Here's how the part is built. I have some questions about the finished solid (model axes, mm). A direction names the side the tool comes from. Coordinates: 2 decimals unless noted, no trailing zeros. Write each loop counter-clockwise with the first axis right and the second up, starting at its lowest first coordinate (ties: lowest second). Pieces come first, ordered by that corner, then holes. Notation, with made-up numbers: (59, 18.25) -> (67, 18.25) arc R17 ccw to (67, 34.25) -> close; hole circle Ø10 at (31.5, 13). An arc over 180 degrees is marked (long way). Put each result on its own line as item: value.
```python
from build123d import *

# Parameters (mm, degrees)
PAD_DEPTH            = 31
FILLET_R             = 15
POCKET_DEPTH         = 24.023168
FILLET001_R          = 15
POCKET001_DEPTH      = 18.144337
POCKET001_DEPTH_BACK = -16.633037
FILLET002_R          = 10
SKETCH003_R          = 7.670171
POCKET002_DEPTH      = 18.144337
POCKET002_DEPTH_BACK = -16.633037
POCKET003_DEPTH      = 18.144337
POCKET003_DEPTH_BACK = -16.633037


with BuildPart() as part:
    # Sketch → Pad (new body)
    with BuildSketch(Plane.XY):
        with BuildLine():
            Line((17.5802, 5.874869), (-57.733299, 5.874869))
            Line((-57.733299, 5.874869), (-57.733299, -5.878831))
            Line((-57.733299, -5.878831), (17.914803, -5.878831))
            ThreePointArc((24.661976, -7.143267), (21.347118, -6.197668), (17.914803, -5.878831))
            Line((24.661976, -7.143267), (45.314852, -15.165812))
            ThreePointArc((45.314852, -15.165812), (49.158723, -16.262318), (53.138796, -16.632037))
            Line((53.138796, -16.632037), (98.306877, -16.632037))
            Line((98.306877, -16.632037), (98.306877, -11.884055))
            Line((98.306877, -11.884055), (53.335909, -11.884055))
            ThreePointArc((45.371277, -10.225885), (49.268204, -11.465115), (53.335909, -11.884055))
            Line((32.389291, -4.575495), (45.371277, -10.225885))
            ThreePointArc((32.39346, 4.595455), (29.384719, 0.011347), (32.389291, -4.575495))
            Line((44.784154, 9.975093), (32.39346, 4.595455))
            ThreePointArc((53.974339, 11.884055), (49.281162, 11.401775), (44.784154, 9.975093))
            Line((98.300218, 11.884055), (53.974339, 11.884055))
            Line((98.300218, 18.143337), (98.300218, 11.884055))
            Line((53.605767, 18.143337), (98.300218, 18.143337))
            ThreePointArc((53.605767, 18.143337), (50.367046, 17.81052), (47.2637, 16.825979))
            Line((26.131771, 7.651179), (47.2637, 16.825979))
            ThreePointArc((17.5802, 5.874869), (21.947254, 6.323636), (26.131771, 7.651179))
        make_face()
    extrude(amount=PAD_DEPTH)

    # Fillet
    fillet_edges = [part.edges().sort_by_distance(p)[0] for p in [
        (98.306877, -14.258046, 31),
        (98.300218, 15.013696, 31),
        (98.306877, -14.258046, 0),
        (98.300218, 15.013696, 0),
    ]]
    fillet(fillet_edges, radius=FILLET_R)

    # Sketch001 (on Face13 of Fillet) → Pocket (cut, through all)
    with BuildSketch(Plane(origin=(3, -5.878831, 20), x_dir=(0.891007, 0, 0.45399), z_dir=(0, -1, 0))):
        with BuildLine():
            ThreePointArc((-28.331719, 19.051588), (-53.844012, 15.55741), (-28.331719, 12.063232))
            Line((-25.207983, 12.063232), (-28.331719, 12.063232))
            Line((-25.207983, 19.051588), (-25.207983, 12.063232))
            Line((-28.331719, 19.051588), (-25.207983, 19.051588))
        make_face()
    extrude(amount=-POCKET_DEPTH, mode=Mode.SUBTRACT)

    # Fillet001
    fillet001_edges = [part.edges().sort_by_distance(p)[0] for p in [
        (-57.733299, -0.001981, 31),
        (-57.733299, -0.001981, 0),
    ]]
    fillet(fillet001_edges, radius=FILLET001_R)

    # Sketch002 → Pocket001 (cut, two sides)
    with BuildSketch(Plane.XZ) as pocket001_sk:
        Polygon((-48.132477, 32.687893), (93.832344, 26.227839), (93.832344, 4.772161), (-48.132477, -1.687893), (-48.132477, -33.037488), (136.738275, -33.037488), (136.738275, 64.037488), (-48.132477, 64.037488), align=None)
    extrude(amount=-POCKET001_DEPTH, mode=Mode.SUBTRACT)
    extrude(pocket001_sk.sketch, amount=-POCKET001_DEPTH_BACK, mode=Mode.SUBTRACT)

    # Fillet002
    fillet002_edges = [part.edges().sort_by_distance(p)[0] for p in [
        (93.832344, 15.013696, 26.227839),
        (93.832344, -14.258046, 26.227839),
        (93.832344, 15.013696, 4.772161),
        (93.832344, -14.258046, 4.772161),
    ]]
    fillet(fillet002_edges, radius=FILLET002_R)

    # Sketch003 → Pocket002 (cut, two sides)
    with BuildSketch(Plane.XZ) as pocket002_sk:
        with Locations((81.142525, 15.22629)):
            Circle(SKETCH003_R)
    extrude(amount=-POCKET002_DEPTH, mode=Mode.SUBTRACT)
    extrude(pocket002_sk.sketch, amount=-POCKET002_DEPTH_BACK, mode=Mode.SUBTRACT)

    # Sketch004 → Pocket003 (cut, two sides)
    with BuildSketch(Plane.XZ) as pocket003_sk:
        with BuildLine():
            ThreePointArc((-15.271182, 25.376072), (-18.898724, 23.62511), (-19.082655, 19.601294))
            ThreePointArc((-18.766414, 9.83565), (-17.972747, 14.749294), (-19.082655, 19.601294))
            ThreePointArc((-18.766414, 9.83565), (-19.039764, 5.656397), (-15.390545, 3.601138))
            Line((-15.390545, 3.601138), (55.165915, 7.037659))
            ThreePointArc((55.165915, 7.037659), (63.138146, 15.614512), (54.086796, 23.043639))
            Line((-15.271182, 25.376072), (54.086796, 23.043639))
        make_face()
    extrude(amount=-POCKET003_DEPTH, mode=Mode.SUBTRACT)
    extrude(pocket003_sk.sketch, amount=-POCKET003_DEPTH_BACK, mode=Mode.SUBTRACT)


solid = part.part
```
Item 1: Imagine slicing it at D-D on x = 40.5. Write out the boundary of the cut face in (y, z).
Output:
outline: (-13.3, 2.35) -> (-8.11, 2.35) -> (-8.11, 6.32) -> (-13.3, 6.32) -> close; (-13.3, 23.5) -> (-8.11, 23.5) -> (-8.11, 28.65) -> (-13.3, 28.65) -> close; (8.12, 2.35) -> (13.89, 2.35) -> (13.89, 6.32) -> (8.12, 6.32) -> close; (8.12, 23.5) -> (13.89, 23.5) -> (13.89, 28.65) -> (8.12, 28.65) -> close
Item 2: For P1, Ø8, axis at y = -12.5, z = 22.5, coming from the +X side; P2, Ø15.5, axis at x = -25.5, z = 14, coming from the -Y side; P3, Ø12, axis at x = 12, y = 0.5, coming from the +Z side, each with a flat end and sliding along its axis, tell me the tip position at first contact or that it passes through.
Output:
P1: stops at x = 93.66
P2: stops at y = -5.88
P3: stops at z = 30.22
Item 3: Imagine slicing it at B-B on x = -4. Write out the boundary of the cut face in (y, z), then the cut area to 3 significant figures.
Output:
outline: (-5.88, 0.32) -> (5.87, 0.32) -> (5.87, 4.16) -> (-5.88, 4.16) -> close; (-5.88, 25) -> (5.87, 25) -> (5.87, 30.68) -> (-5.88, 30.68) -> close
area: 112 mm²
Item 4: Imagine slicing it at C-C on y = 14.5. Write out the boundary of the cut face in (x, z), then the cut area to 3 significant figures.
Output:
outline: (41.91, 2.41) -> (84.29, 4.34) arc R10 ccw to (93.83, 14.33) -> (93.83, 16.67) arc R10 ccw to (84.29, 26.66) -> (41.91, 28.59) -> (41.91, 23.45) -> (54.09, 23.04) arc R8.04 cw (long way) to (55.17, 7.04) -> (41.91, 6.39) -> close; hole circle Ø15.34 at (81.14, 15.23)
area: 694 mm²
Item 5: Please list where these lines run through material, in increasing order: line 1 along X through (y, z) = (-5, 15); line 2 along Y through (x, z) = (45.5, 23.5); line 3 along Z through (x, y) = (80.5, -14). Write a range as from..to.
Output:
line 1: x = -57.73..-53.45, -27.47..-17.98
line 2: y = -15.24..-10.28, 10.27..16.06
line 3: z = 4.17..7.58, 22.87..26.83
Item 6: Which directions (+Z, -Z, +X, -X, +Y, -Y) give clear straight access to the entire face, cutting with the end or side of a thin tool? Please do faces 4 (the flat face through (73, 18.143, 15)), 5 (the flat face through (38.79, -7.36, 26.14)), 6 (the flat face through (-20, 5.875, 15)).
Output:
face 4: +Z, -Z, +X, -X, +Y
face 5: +Z, -Z, +X
face 6: +Z, -Z, -X, +Y
Item 7: Imagine slicing it at A-A on x = 77.5. Write out the boundary of the cut face in (y, z), then the cut area to 3 significant figures.
Output:
outline: (-16.63, 4.03) -> (-11.88, 4.03) -> (-11.88, 8.48) -> (-16.63, 8.48) -> close; (-16.63, 21.98) -> (-11.88, 21.98) -> (-11.88, 26.97) -> (-16.63, 26.97) -> close; (11.88, 4.03) -> (18.14, 4.03) -> (18.14, 8.48) -> (11.88, 8.48) -> close; (11.88, 21.98) -> (18.14, 21.98) -> (18.14, 26.97) -> (11.88, 26.97) -> close
area: 104 mm²
Item 8: If we mould it in two halves opening along X, with no side actions, what happens to faces 1 (the cylindrical face through (-52.266, -0.084, 9.887)), 2 (the flat face through (32.9, -5.8, 29)), 3 (the flat face through (73.87, -11.884, 18.12))? For each: released by +X, released by -X, zero draft, split by the parting line, or undercut.
Output:
face 1: undercut
face 2: released by +X
face 3: zero draft
